For this review, take the finished solid that the model builds, in its own axes (mm). A direction names the side the tool comes from. Round coordinates to 2 decimals unless told otherwise and drop trailing zeros. Loops run counter-clockwise (first coordinate to the right, second up) from the corner with the lowest first, then second, coordinate; pieces in that order, holes last. Notation, with made-up numbers: (8.25, 82.5) -> (14.25, 82.5) arc R22 ccw to (14.25, 95.5) -> close; hole circle Ø11 at (62, 88.25). An arc over 180 degrees is marked (long way). One line per question, with ' | ' between items. Start each with the question number.
1. Consider section A-A (z = -3.25). Write out the cut boundary in (x, y).
2. For pin 1 Ø4 at (x, z) = (85, -5.5) entering from -Y; pin 2 Ø3 at (x, z) = (26, -8.5) entering from -Y; pin 3 Ø1.5 at (y, z) = (-2, -5.5) entering from +X; pin 4 Ø1 at (y, z) = (-10.5, -10.5) entering from -X, all flat-tipped, find the tip position at first contact; note any pin that passes through.
3. Wall thickness on line 1 along Z through (x, y) = (81.5, -8.5); line 2 along X through (y, z) = (-5.75, -9.25); line 3 along X through (y, z) = (-11, -2.75): over which ranges is each line inside the solid? List them lowest first.
4. For faces 4 (the face through (-6.35, -6.49, -6.26)), 5 (the face through (82, -6.35, -6)), 6 (the face through (89.526, -6, -10)), 7 (the face through (97, -3, -10.16)), list the 3-axis set-ups (+Z, -Z, +X, -X, +Y, -Y) from which the entire face can be reached by the end or side of a thin tool; tool diameter is ignored.
5. Draft analysis for pull direction Y (two halves, no side actions). For faces 1 (the face through (55, -12.7, -6)), 2 (the face through (30.542, -9.569, -8.694)), 3 (the face through (97.38, -3.05, -8.28)), state which applies: pulls with the +Y half, pulls with the -Y half, needs draft (parallel to the pull), parting line crosses it, or undercut.
```python
from build123d import *

# Parameters (mm, degrees)
BOSS_EXTRUDE1_DEPTH = 12.7
CUT_EXTRUDE1_DEPTH  = 6.35
CUT_EXTRUDE4_START  = 3.81
CUT_EXTRUDE4_DEPTH  = 3.81
CUT_EXTRUDE5_DEPTH  = 5.08
SKETCH5_R           = 5.08
CUT_EXTRUDE6_DEPTH  = 6.35


# Read off the part's stored shape, not the designer's step: Cut-Extrude5
with BuildPart() as part:
    # Sketch1 → Boss-Extrude1 (new body)
    with BuildSketch(Plane.XY):
        with BuildLine():
            Line((0, 0), (107.95, 0))
            ThreePointArc((107.95, 0), (114.3, -6.35), (107.95, -12.7))
            Line((107.95, -12.7), (0, -12.7))
            ThreePointArc((0, -12.7), (-6.35, -6.35), (0, 0))
        make_face()
    extrude(amount=-BOSS_EXTRUDE1_DEPTH)

    # Sketch2 → Cut-Extrude1 (cut)
    with BuildSketch(Plane(origin=(0, 0, -12.7), x_dir=(-1, 0, 0), z_dir=(0, 0, -1))):
        with BuildLine():
            Line((-98.543781691, -5.269443984), (-97.020546117, -5.269443984))
            ThreePointArc((-97.020546117, -5.269443984), (-94.03507736, -3.175), (-91.049608603, -5.269443984))
            Line((-91.049608603, -5.269443984), (-89.526373029, -5.269443984))
            Line((-89.526373029, -5.269443984), (-89.526373029, -7.430556016))
            Line((-89.526373029, -7.430556016), (-91.049608603, -7.430556016))
            ThreePointArc((-91.049608603, -7.430556016), (-94.03507736, -9.525), (-97.020546117, -7.430556016))
            Line((-97.020546117, -7.430556016), (-98.543781691, -7.430556016))
            Line((-98.543781691, -7.430556016), (-98.543781691, -5.269443984))
        make_face()
        with BuildLine():
            Line((-18.423626971, -5.269443984), (-18.423626971, -7.430556016))
            Line((-18.423626971, -7.430556016), (-16.900391397, -7.430556016))
            ThreePointArc((-16.900391397, -7.430556016), (-13.91492264, -9.525), (-10.929453883, -7.430556016))
            Line((-10.929453883, -7.430556016), (-9.406218309, -7.430556016))
            Line((-9.406218309, -7.430556016), (-9.406218309, -5.269443984))
            Line((-9.406218309, -5.269443984), (-10.929453883, -5.269443984))
            ThreePointArc((-10.929453883, -5.269443984), (-13.91492264, -3.175), (-16.900391397, -5.269443984))
            Line((-16.900391397, -5.269443984), (-18.423626971, -5.269443984))
        make_face()
    extrude(amount=-CUT_EXTRUDE1_DEPTH, mode=Mode.SUBTRACT)

    # Sketch3 → Cut-Extrude4 (cut)
    with BuildSketch(Plane(origin=(0, 0, -6.35), x_dir=(-1, 0, 0), z_dir=(0, 0, -1)).offset(CUT_EXTRUDE4_START)):
        with BuildLine():
            ThreePointArc((-14.99442264, -1.777413667), (-11.444937607, -2.353371426), (-9.342336307, -5.2705))
            Line((-9.342336307, -5.2705), (-10.929071882, -5.2705))
            ThreePointArc((-10.929071882, -5.2705), (-12.566929092, -3.475362911), (-14.99442264, -3.364149242))
            Line((-14.99442264, -3.364149242), (-14.99442264, -1.777413667))
        make_face()
        with BuildLine():
            ThreePointArc((-12.834322649, -10.922326506), (-16.383098929, -10.347745843), (-18.486790701, -7.432537968))
            Line((-18.486790701, -7.432537968), (-16.900008973, -7.431612032))
            ThreePointArc((-16.900008973, -7.431612032), (-15.26155345, -9.225275719), (-12.834704368, -9.335590978))
            Line((-12.834704368, -9.335590978), (-12.834322649, -10.922326506))
        make_face()
        with BuildLine():
            ThreePointArc((-95.115295632, -9.335590978), (-92.68844655, -9.225275719), (-91.049991027, -7.431612032))
            Line((-91.049991027, -7.431612032), (-89.463209299, -7.432537968))
            ThreePointArc((-89.463209299, -7.432537968), (-91.566901071, -10.347745843), (-95.115677351, -10.922326506))
            Line((-95.115677351, -10.922326506), (-95.115295632, -9.335590978))
        make_face()
        with BuildLine():
            ThreePointArc((-92.95557736, -3.364149242), (-95.383070908, -3.475362911), (-97.020928118, -5.2705))
            Line((-97.020928118, -5.2705), (-98.607663693, -5.2705))
            ThreePointArc((-98.607663693, -5.2705), (-96.505062393, -2.353371426), (-92.95557736, -1.777413667))
            Line((-92.95557736, -1.777413667), (-92.95557736, -3.364149242))
        make_face()
    extrude(amount=-CUT_EXTRUDE4_DEPTH, mode=Mode.SUBTRACT)

    # Cut-Extrude5 outline → Cut-Extrude5 (cut)
    with BuildSketch(Plane(origin=(0, 0, -6.35), x_dir=(-1, 0, 0), z_dir=(0, 0, -1))):
        with BuildLine():
            ThreePointArc((-9.342336307, -5.2705), (-11.444937607, -2.353371426), (-14.99442264, -1.777413667))
            Line((-14.99442264, -1.777413667), (-14.99442264, -3.364149242))
            ThreePointArc((-14.99442264, -3.364149242), (-12.567437486, -3.475124566), (-10.929453883, -5.269443984))
            Line((-10.929453883, -5.269443984), (-9.406218309, -5.269443984))
            Line((-9.406218309, -5.269443984), (-9.406218309, -5.2705))
            Line((-9.406218309, -5.2705), (-9.342336307, -5.2705))
        make_face()
        with BuildLine():
            ThreePointArc((-18.486790701, -7.432537968), (-16.383098929, -10.347745843), (-12.834322649, -10.922326506))
            Line((-12.834322649, -10.922326506), (-12.834704368, -9.335590978))
            ThreePointArc((-12.834704368, -9.335590978), (-12.835063496, -9.335720889), (-12.83542264, -9.335850758))
            Line((-12.83542264, -9.335850758), (-12.83542264, -10.796172665))
            Line((-12.83542264, -10.796172665), (-14.99442264, -10.796172665))
            Line((-14.99442264, -10.796172665), (-14.99442264, -9.335850758))
            ThreePointArc((-14.99442264, -9.335850758), (-16.159192409, -8.595858011), (-16.900008973, -7.431612032))
            Line((-16.900008973, -7.431612032), (-18.486790701, -7.432537968))
        make_face()
        with BuildLine():
            ThreePointArc((-95.11457736, -3.364149242), (-94.03507736, -3.175), (-92.95557736, -3.364149242))
            Line((-92.95557736, -3.364149242), (-92.95557736, -1.651))
            Line((-92.95557736, -1.651), (-95.11457736, -1.651))
            Line((-95.11457736, -1.651), (-95.11457736, -3.364149242))
        make_face()
        with BuildLine():
            Line((-92.95557736, -10.796172665), (-92.95557736, -9.335850758))
            ThreePointArc((-92.95557736, -9.335850758), (-94.03507736, -9.525), (-95.11457736, -9.335850758))
            Line((-95.11457736, -9.335850758), (-95.11457736, -10.796172665))
            Line((-95.11457736, -10.796172665), (-92.95557736, -10.796172665))
        make_face()
    extrude(amount=CUT_EXTRUDE5_DEPTH, mode=Mode.SUBTRACT)

    # Sketch5 → Cut-Extrude6 (cut)
    with BuildSketch(Plane(origin=(0, -12.7, 0), x_dir=(1, 0, 0), z_dir=(0, 1, 0))):
        with Locations(Location((81.915, 6.35, 0), (0, 0, 270))):
            Circle(SKETCH5_R)
        with Locations(Location((26.035, 6.35, 0), (0, 0, 90))):
            Circle(SKETCH5_R)
    extrude(amount=CUT_EXTRUDE6_DEPTH, mode=Mode.SUBTRACT)


solid = part.part
```
Answer block:
1) outline: (0, -12.7) -> (22.01, -12.7) -> (22.01, -6.35) -> (30.06, -6.35) -> (30.06, -12.7) -> (77.89, -12.7) -> (77.89, -6.35) -> (85.94, -6.35) -> (85.94, -12.7) -> (107.95, -12.7) arc R6.35 ccw to (107.95, 0) -> (0, 0) arc R6.35 ccw to start
2) pin 1: stops at y = -12.7 | pin 2: stops at y = -6.35 | pin 3: stops at x = 113.18 | pin 4: stops at x = -5.2
3) line 1: z = -12.7 to -11.41, -1.29 to 0 | line 2: x = -6.32 to 9.41, 18.42 to 89.53, 98.54 to 114.27 | line 3: x = -4.32 to 22.45, 29.62 to 78.33, 85.5 to 112.27
4) face 4: +Z, -Z, -X | face 5: -Y | face 6: -Z | face 7: none
5) face 1: pulls with the -Y half | face 2: needs draft | face 3: undercut
